from build123d import *

# Parameters (mm, degrees)
SKETCH1_W           = 19.05
SKETCH1_H           = 40
BOSS_EXTRUDE1_DEPTH = 12.7
SKETCH2_W           = 19.05
SKETCH2_H           = 6.35
BOSS_EXTRUDE2_DEPTH = 69.85
CUT_EXTRUDE1_REACH  = 95.688
SKETCH5_R           = 6.35
SKETCH6_R           = 6.35
CUT_EXTRUDE2_DEPTH  = 94.687806037
FILLET4_R           = 3.81


with BuildPart() as part:
    # Sketch1 → Boss-Extrude1 (new body)
    with BuildSketch(Plane(origin=(0, 0, 0), x_dir=(0, 0, -1), z_dir=(1, 0, 0))):
        with Locations((9.525, 20)):
            Rectangle(SKETCH1_W, SKETCH1_H)
    extrude(amount=BOSS_EXTRUDE1_DEPTH)

    # Sketch2 → Boss-Extrude2 (add)
    with BuildSketch(Plane(origin=(12.7, 0, 0), x_dir=(0, 0, -1), z_dir=(1, 0, 0))):
        with Locations((9.525, 3.175)):
            Rectangle(SKETCH2_W, SKETCH2_H)
        with Locations((9.525, 36.825)):
            Rectangle(SKETCH2_W, SKETCH2_H)
    extrude(amount=BOSS_EXTRUDE2_DEPTH)

    # Sketch5 → Cut-Extrude1 (cut, up to next)
    with BuildSketch(Plane.ZY, mode=Mode.PRIVATE) as cut_extrude1_sk1:
        with Locations((-9.525, 20)):
            Circle(SKETCH5_R)
    cut_extrude1_tool1 = extrude(cut_extrude1_sk1.sketch, amount=-CUT_EXTRUDE1_REACH, mode=Mode.PRIVATE) & part.part
    add(cut_extrude1_tool1.solids().sort_by_distance((0, 20, -9.525))[0], mode=Mode.SUBTRACT)

    # Sketch6 → Cut-Extrude2 (cut, through all)
    with BuildSketch(Plane.XZ):
        with Locations(Location((73.1, -9.45, 0), (0, 0, 270))):
            Circle(SKETCH6_R)
    extrude(amount=-CUT_EXTRUDE2_DEPTH, mode=Mode.SUBTRACT)

    # Fillet4
    # the kernel refuses this fillet: 3.81 mm, written as the material it adds along each edge
    with BuildSketch(Plane(origin=(12.7, 33.65, 0), x_dir=(1, 0, 0), z_dir=(0, 0, -1)), Plane(origin=(12.7, 6.35, 0), x_dir=(0, 1, 0), z_dir=(0, 0, -1))) as fillet4_piece_1:
        with BuildLine():
            CenterArc((FILLET4_R, FILLET4_R), FILLET4_R, 180, 90)
            Line((0, FILLET4_R), (0, 0))
            Line((0, 0), (FILLET4_R, 0))
        make_face()
    extrude(amount=19.05)
    # the kernel refuses this fillet: 3.81 mm, written as the material it takes off along each edge
    with BuildSketch(Plane(origin=(0, 0, 9.525), x_dir=(1, 0, 0), z_dir=(0, 0, -1)), Plane(origin=(82.55, 0, -28.575), x_dir=(-1, 0, 0), z_dir=(0, 0, 1)), Plane(origin=(82.55, 33.65, 9.525), x_dir=(0, 1, 0), z_dir=(0, 0, -1))) as fillet4_2_piece_1:
        with BuildLine():
            CenterArc((FILLET4_R, -FILLET4_R), FILLET4_R, 90, 90)
            Line((0, -FILLET4_R), (0, 0))
            Line((0, 0), (FILLET4_R, 0))
        make_face()
    extrude(amount=38.1, mode=Mode.SUBTRACT)
    with BuildSketch(Plane(origin=(0, 40, -28.575), x_dir=(0, -1, 0), z_dir=(0, 0, 1)), Plane(origin=(82.55, 6.35, 9.525), x_dir=(0, -1, 0), z_dir=(0, 0, -1)), Plane(origin=(82.55, 40, -28.575), x_dir=(-1, 0, 0), z_dir=(0, 0, 1))) as fillet4_2_piece_2:
        with BuildLine():
            CenterArc((FILLET4_R, FILLET4_R), FILLET4_R, 180, 90)
            Line((0, FILLET4_R), (0, 0))
            Line((0, 0), (FILLET4_R, 0))
        make_face()
    extrude(amount=38.1, mode=Mode.SUBTRACT)


solid = part.part
Model file for the job. Use its own axes, mm. A direction names the side the tool comes from. Give positions to 0.01 mm unless a question says otherwise; leave off trailing zeros. Loops run counter-clockwise (first coordinate to the right, second up) from the corner with the lowest first, then second, coordinate; pieces in that order, holes last.
Item 1: Mould opens along Z. For faces 1 (the face through (79.396, 36.781, -8.623)), 2 (the face through (32, 5, 0)), 3 (the face through (12.7, 20, -3)) say: +Z half, -Z half, draft (parallel to the pull), parting line (faces both ways), or undercut.
Check values:
face 1: undercut
face 2: +Z half
face 3: draft
Item 2: Drop flat-ended pins along their axis: P1, Ø4, axis at x = 68.5, z = -3.5, coming from the -Y side; P2, Ø3, axis at y = 17.5, z = -4.5, coming from the +X side. Give the stop position or say it passes through.
Check values:
P1: stops at y = 0
P2: stops at x = 12.7
Item 3: Which spindle directions (+Z, -Z, +X, -X, +Y, -Y) get a long thin tool onto all of the face, cutting with end or side? Do faces 4 (the face through (47, 33.65, -9)), 5 (the face through (1.146, 1.086, -9.392)). Say none if no direction does.
Check values:
face 4: +Z, -Z, +X
face 5: +Z, -Z, -X, -Y
Item 4: Slice it at D-D (x = 73.1). Write the cut outline in (y, z), plus the area to 3 significant figures.
Check values:
outline: (0, -19.05) - (6.35, -19.05) - (6.35, -15.8) - (0, -15.8) - close; (0, -3.1) - (6.35, -3.1) - (6.35, 0) - (0, 0) - close; (33.65, -19.05) - (40, -19.05) - (40, -15.8) - (33.65, -15.8) - close; (33.65, -3.1) - (40, -3.1) - (40, 0) - (33.65, 0) - close
area: 80.6 mm2
Item 5: Slice it at C-C (z = -11.25). Write the cut outline in (x, y) (3 decimals).
Check values:
outline: (0, 3.81) arc R3.81 ccw to (3.81, 0) - (67.01, 0) - (67.01, 6.35) - (16.51, 6.35) arc R3.81 cw to (12.7, 10.16) - (12.7, 13.889) - (0, 13.889) - close; (0, 26.111) - (12.7, 26.111) - (12.7, 29.84) arc R3.81 cw to (16.51, 33.65) - (67.01, 33.65) - (67.01, 40) - (3.81, 40) arc R3.81 ccw to (0, 36.19) - close; (79.19, 0.027) arc R3.81 ccw to (82.497, 3.175) arc R3.81 ccw to (79.19, 6.323) - close; (79.19, 33.677) arc R3.81 ccw to (82.497, 36.825) arc R3.81 ccw to (79.19, 39.973) - close
Item 6: Slice it at A-A (x = 47.5). Write the cut outline in (y, z).
Check values:
outline: (0, -19.05) - (6.35, -19.05) - (6.35, 0) - (0, 0) - close; (33.65, -19.05) - (40, -19.05) - (40, 0) - (33.65, 0) - close
Item 7: Slice it at B-B (y = 20). Write the cut outline in (x, z) (3 decimals), plus the area to 3 significant figures.
Check values:
outline: (0, -19.05) - (12.7, -19.05) - (12.7, -15.875) - (0, -15.875) - close; (0, -3.175) - (12.7, -3.175) - (12.7, 0) - (0, 0) - close
area: 80.6 mm2
Item 8: Drill centre lines: line 1 along Y through (x, z) = (24, -17); line 2 along X through (y, z) = (28, -17.5). Where is each one in solid material? Low to high.
Check values:
line 1: y = 0 to 6.35, 33.65 to 40
line 2: x = 0 to 12.7
